Input: part model. Units: mm. Frame: model coordinates. Face numbers are marked on the shaded views. Coordinates: 2 decimals unless noted, no trailing zeros. Loops run counter-clockwise (first coordinate to the right, second up) from the corner with the lowest first, then second, coordinate; pieces in that order, holes last.
Item 1: Ray query, line 1 along X through (y, z) = (-3.25, 8); line 2 along Z through (x, y) = (-18, 0.95); line 3 along X through (y, z) = (-4.5, 8.5). Return the intervals inside material, ascending.
Item 2: Section B-B on z = 11.5. Give the number of separate pieces and of enclosed holes in the cut face, and give its area (3 significant figures).
Item 3: Section A-A on x = 36. Return loops of the section in (y, z).
Item 4: Contact query for flat-ended pins moving along their axis: P1, Ø0.9, axis at x = 64.5, z = 11.5, coming from the +Y side; P2, Ø8.5, axis at x = -54, z = 10, coming from the -Y side; P3, Ø9.5, axis at x = 0, z = 10, coming from the -Y side; P4, Ø6.5, axis at x = 54, z = 10, coming from the -Y side. Output: stop coordinate, or through.
Item 5: Section C-C on x = -9.5. Return loops of the section in (y, z), and give its area (3 significant figures).
Item 6: Pull-direction query (X, two-part tool) for the marked faces 1, 2, 3 and 4; classes: released by +X, released by -X, zero draft, split by the parting line, or undercut.
```python
from build123d import *

# Parameters (mm, degrees)
F1_DEPTH     = 20
F2_T4_DEPTH  = 20
F2_T9_DEPTH  = 20
F2_T14_DEPTH = 20
F2_T19_DEPTH = 20
F3_SIZE2     = 1.5
F3_SIZE      = 10
F3_2_SIZE2   = 1.5
F3_2_SIZE    = 10
F3_3_SIZE2   = 1.5
F3_3_SIZE    = 10
F3_4_SIZE2   = 1.5
F3_4_SIZE    = 10
F4_T1_DEPTH  = 14.8584149398
F4_T3_DEPTH  = 14.8584149398
F5_R         = 3.6
F6_DEPTH     = 25
F7_SIZE      = 1


# Not quite as in the source:
# - a fillet or chamfer that OpenCascade refuses, or shapes differently, is made with other operations: its cross-section is extruded or revolved along the edge and cut away or added


with BuildPart() as f1:
    # F0 (on Top) → F1 (new body)
    with BuildSketch(Plane.XY):
        Polygon((-70, 6), (-70, 0), (-70, -6), (-66.5, -6), (-66.5, -4), (-68, -4), (-68, -1.9), (-65, -1.9), (-65, -2.9), (-64, -2.9), (-64, -2.5), (0, -2.5), (64, -2.5), (64, -2.9), (65, -2.9), (65, -1.9), (68, -1.9), (68, -4), (66.5, -4), (66.5, -6), (70, -6), (70, 0), (70, 6), (66.5, 6), (66.5, 4), (68, 4), (68, 1.9), (65, 1.9), (65, 2.9), (64, 2.9), (64, 2.5), (0, 2.5), (-64, 2.5), (-64, 2.9), (-65, 2.9), (-65, 1.9), (-68, 1.9), (-68, 4), (-66.5, 4), (-66.5, 6), align=None)
    extrude(amount=F1_DEPTH)

    # F2: chamfer of 0.5 on 4 edges, made by hand


with BuildPart() as f2_tool2:
    # F2_s3 → F2_t4 (new body)
    with BuildSketch(Plane.XY):
        Polygon((-64, 3), (-63.5, 2.5), (-64, 2.5), align=None)
    extrude(amount=F2_T4_DEPTH)

    split(bisect_by=Plane.XZ.offset(-2.9), keep=Keep.TOP)


with BuildPart() as f1_1:
    add(f1.part)

    # F2_t1: union F2_tool2
    add(f2_tool2.part)


with BuildPart() as f2_tool7:
    # F2_s8 → F2_t9 (new body)
    with BuildSketch(Plane.XY):
        Polygon((-63.5, -2.5), (-64, -3), (-64, -2.5), align=None)
    extrude(amount=F2_T9_DEPTH)

    split(bisect_by=Plane.XZ.offset(2.9), keep=Keep.BOTTOM)


with BuildPart() as f1_2:
    add(f1_1.part)

    # F2_t6: union F2_tool7
    add(f2_tool7.part)


with BuildPart() as f2_tool12:
    # F2_s13 → F2_t14 (new body)
    with BuildSketch(Plane.XY):
        Polygon((64, -3), (63.5, -2.5), (64, -2.5), align=None)
    extrude(amount=F2_T14_DEPTH)

    split(bisect_by=Plane.XZ.offset(2.9), keep=Keep.BOTTOM)


with BuildPart() as f1_3:
    add(f1_2.part)

    # F2_t11: union F2_tool12
    add(f2_tool12.part)


with BuildPart() as f2_tool17:
    # F2_s18 → F2_t19 (new body)
    with BuildSketch(Plane.XY):
        Polygon((63.5, 2.5), (64, 3), (64, 2.5), align=None)
    extrude(amount=F2_T19_DEPTH)

    split(bisect_by=Plane.XZ.offset(-2.9), keep=Keep.TOP)


with BuildPart() as f1_4:
    add(f1_3.part)

    # F2_t16: union F2_tool17
    add(f2_tool17.part)

    # F3
    f3_edges = [f1_4.edges().sort_by_distance(p)[0] for p in [
        (-66.5, 5, 20),
    ]]
    f3_side = f1_4.faces().sort_by_distance((-66.5, 5, 10))[0]
    chamfer(f3_edges, length=F3_SIZE, length2=F3_SIZE2, reference=f3_side)

    # F3#2
    f3_2_edges = [f1_4.edges().sort_by_distance(p)[0] for p in [
        (-66.5, -5, 20),
    ]]
    f3_2_side = f1_4.faces().sort_by_distance((-66.5, -5, 10))[0]
    chamfer(f3_2_edges, length=F3_2_SIZE, length2=F3_2_SIZE2, reference=f3_2_side)

    # F3#3
    f3_3_edges = [f1_4.edges().sort_by_distance(p)[0] for p in [
        (66.5, 5, 20),
    ]]
    f3_3_side = f1_4.faces().sort_by_distance((66.5, 5, 10))[0]
    chamfer(f3_3_edges, length=F3_3_SIZE, length2=F3_3_SIZE2, reference=f3_3_side)

    # F3#4
    f3_4_edges = [f1_4.edges().sort_by_distance(p)[0] for p in [
        (66.5, -5, 20),
    ]]
    f3_4_side = f1_4.faces().sort_by_distance((66.5, -5, 10))[0]
    chamfer(f3_4_edges, length=F3_4_SIZE, length2=F3_4_SIZE2, reference=f3_4_side)

    # F4: chamfer of 2.5 on 4 edges, made by hand

    # F4_s2 → F4_t1 (cut)
    with BuildSketch(Plane.YZ.offset(-76.4292074699)):
        Polygon((3.5, 20), (6, 17.5), (6, 20), align=None)
        Polygon((-3.5, 20), (-6, 17.5), (-6, 20), align=None)
    extrude(amount=F4_T1_DEPTH, mode=Mode.SUBTRACT)

    # F4_s4 → F4_t3 (cut)
    with BuildSketch(Plane.YZ.offset(61.5707925301)):
        Polygon((3.5, 20), (6, 17.5), (6, 20), align=None)
        Polygon((-3.5, 20), (-6, 17.5), (-6, 20), align=None)
    extrude(amount=F4_T3_DEPTH, mode=Mode.SUBTRACT)

    # F5 (on face) → F6 (cut)
    with BuildSketch(Plane.XZ.offset(2.5)):
        with Locations((-54, 10)):
            Circle(F5_R)
        with Locations((-36, 10)):
            Circle(F5_R)
        with Locations((-18, 10)):
            Circle(F5_R)
        with Locations((0, 10)):
            Circle(F5_R)
        with Locations((18, 10)):
            Circle(F5_R)
        with Locations((36, 10)):
            Circle(F5_R)
        with Locations((54, 10)):
            Circle(F5_R)
    extrude(amount=-F6_DEPTH, mode=Mode.SUBTRACT)

    # F7
    f7_edges = [f1_4.edges().sort_by_distance(p)[0] for p in [
        (-57.6, -2.5, 10),
        (-50.4, 0, 10),
        (-57.6, 2.5, 10),
        (-39.6, -2.5, 10),
        (-32.4, 0, 10),
        (-39.6, 2.5, 10),
        (-21.6, -2.5, 10),
        (-14.4, 0, 10),
        (-21.6, 2.5, 10),
        (-3.6, -2.5, 10),
        (3.6, 0, 10),
        (-3.6, 2.5, 10),
        (14.4, -2.5, 10),
        (21.6, 0, 10),
        (14.4, 2.5, 10),
        (32.4, -2.5, 10),
        (39.6, 0, 10),
        (32.4, 2.5, 10),
        (50.4, -2.5, 10),
        (57.6, 0, 10),
        (50.4, 2.5, 10),
    ]]
    chamfer(f7_edges, length=F7_SIZE)


solid = f1_4.part
```
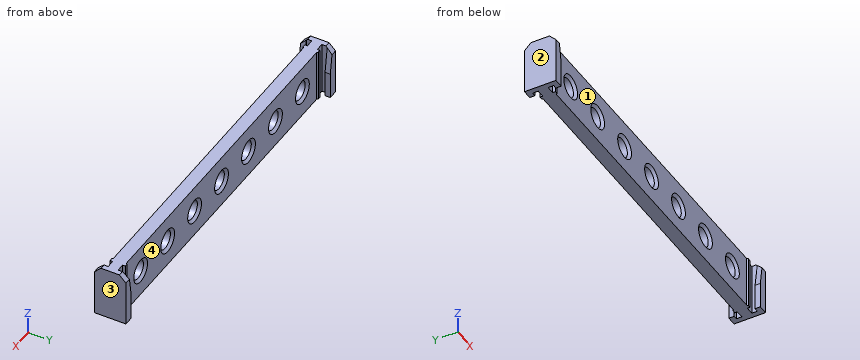
Results found:
1. line 1: x = -70 to -68, 68 to 70
1. line 2: z = 0 to 6.4, 13.6 to 20
1. line 3: x = -70 to -66.5, 66.5 to 70
2. separate pieces: 8
2. enclosed holes: 0
2. area: 489 mm2
3. outline: (-2.5, 0) - (2.5, 0) - (2.5, 5.4) - (1.5, 6.4) - (-1.5, 6.4) - (-2.5, 5.4) - close; (-2.5, 14.6) - (-1.5, 13.6) - (1.5, 13.6) - (2.5, 14.6) - (2.5, 20) - (-2.5, 20) - close
4. P1: stops at y = 2.9
4. P2: stops at y = -2.15
4. P3: stops at y = -2.5
4. P4: passes through
5. outline: (-2.5, 0) - (2.5, 0) - (2.5, 20) - (-2.5, 20) - close
5. area: 100 mm2
6. face 1: undercut
6. face 2: released by -X
6. face 3: released by +X
6. face 4: undercut
